Geometry check sheet. Reference: the model listing, model coordinates, mm. Round coordinates to 2 decimals unless told otherwise and drop trailing zeros. One line per question, with ' | ' between items.
Autodesk Inventor part; units mm, degrees
ref_plane "Start Plane" through (20, 0, 0) normal (1, 0, 0) x (0, 1, 0)
ref_plane "End Plane" through (220.5, 0, 0) normal (1, 0, 0) x (0, 1, 0)
ref_plane "XZ Plane" through (0, 0, 0) normal (0, 1, 0) x (-1, 0, 0)
ref_plane "Start Plane" through (20, 0, 0) normal (1, 0, 0) x (0, 1, 0)
ref_plane "End Plane" through (220.5, 0, 0) normal (1, 0, 0) x (0, 1, 0)
sketch "Sketch" plane through (0, 0, 0) normal (1, 0, 0) x (0, 1, 0)
  circle A0 centre (-3.0533, 11.4582) radius 2.1463
  line L0 (2.4543, 4.6976) -> (0.1995, 6.9525)
  arc A1 (1.8616, 3.2667) -> (2.4543, 4.6976) centre (1.8616, 4.1049) ccw
  line L1 (-0.2466, 3.2667) -> (1.8616, 3.2667)
  arc A2 (-0.2466, 3.2667) -> (-0.5514, 2.9619) centre (-0.2466, 2.9619) ccw
  line L2 (-0.5514, 2.2507) -> (-0.5514, 2.9619)
  arc A3 (-0.5514, 2.2507) -> (0.236, 1.4633) centre (0.236, 2.2507) ccw
  line L3 (4.935, 1.4633) -> (0.236, 1.4633)
  arc A4 (4.935, 1.4633) -> (6.9416, 3.4699) centre (4.935, 3.4699) ccw
  line L4 (6.9416, 8.1689) -> (6.9416, 3.4699)
  arc A5 (6.9416, 8.1689) -> (6.1542, 8.9563) centre (6.1542, 8.1689) ccw
  line L5 (5.443, 8.9563) -> (6.1542, 8.9563)
  arc A6 (5.443, 8.9563) -> (5.1382, 8.6515) centre (5.443, 8.6515) ccw
  line L6 (5.1382, 6.5433) -> (5.1382, 8.6515)
  arc A7 (3.7073, 5.9506) -> (5.1382, 6.5433) centre (4.3, 6.5433) ccw
  line L7 (1.4525, 8.2055) -> (3.7073, 5.9506)
  arc A8 (0.5746, 10.3248) -> (1.4525, 8.2055) centre (3.5718, 10.3248) ccw
  line L8 (0.5746, 12.5917) -> (0.5746, 10.3248)
  arc A9 (1.4525, 14.711) -> (0.5746, 12.5917) centre (3.5718, 12.5917) ccw
  line L9 (3.7073, 16.9658) -> (1.4525, 14.711)
  arc A10 (5.1382, 16.3731) -> (3.7073, 16.9658) centre (4.3, 16.3731) ccw
  line L10 (5.1382, 14.2649) -> (5.1382, 16.3731)
  arc A11 (5.1382, 14.2649) -> (5.443, 13.9601) centre (5.443, 14.2649) ccw
  line L11 (6.1542, 13.9601) -> (5.443, 13.9601)
  arc A12 (6.1542, 13.9601) -> (6.9416, 14.7475) centre (6.1542, 14.7475) ccw
  line L12 (6.9416, 19.4465) -> (6.9416, 14.7475)
  arc A13 (6.9416, 19.4465) -> (4.935, 21.4531) centre (4.935, 19.4465) ccw
  line L13 (0.236, 21.4531) -> (4.935, 21.4531)
  arc A14 (0.236, 21.4531) -> (-0.5514, 20.6657) centre (0.236, 20.6657) ccw
  line L14 (-0.5514, 19.9545) -> (-0.5514, 20.6657)
  arc A15 (-0.5514, 19.9545) -> (-0.2466, 19.6497) centre (-0.2466, 19.9545) ccw
  line L15 (1.8616, 19.6497) -> (-0.2466, 19.6497)
  arc A16 (2.4543, 18.2188) -> (1.8616, 19.6497) centre (1.8616, 18.8115) ccw
  line L16 (0.1995, 15.964) -> (2.4543, 18.2188)
  arc A17 (-1.9199, 15.0861) -> (0.1995, 15.964) centre (-1.9199, 18.0833) ccw
  line L17 (-4.1867, 15.0861) -> (-1.9199, 15.0861)
  arc A18 (-6.306, 15.964) -> (-4.1867, 15.0861) centre (-4.1867, 18.0833) ccw
  line L18 (-8.5609, 18.2188) -> (-6.306, 15.964)
  arc A19 (-7.9682, 19.6497) -> (-8.5609, 18.2188) centre (-7.9682, 18.8115) ccw
  line L19 (-5.86, 19.6497) -> (-7.9682, 19.6497)
  arc A20 (-5.86, 19.6497) -> (-5.5552, 19.9545) centre (-5.86, 19.9545) ccw
  line L20 (-5.5552, 20.6657) -> (-5.5552, 19.9545)
  arc A21 (-5.5552, 20.6657) -> (-6.3426, 21.4531) centre (-6.3426, 20.6657) ccw
  line L21 (-11.0416, 21.4531) -> (-6.3426, 21.4531)
  arc A22 (-11.0416, 21.4531) -> (-13.0482, 19.4465) centre (-11.0416, 19.4465) ccw
  line L22 (-13.0482, 14.7475) -> (-13.0482, 19.4465)
  arc A23 (-13.0482, 14.7475) -> (-12.2608, 13.9601) centre (-12.2608, 14.7475) ccw
  line L23 (-11.5496, 13.9601) -> (-12.2608, 13.9601)
  arc A24 (-11.5496, 13.9601) -> (-11.2448, 14.2649) centre (-11.5496, 14.2649) ccw
  line L24 (-11.2448, 16.3731) -> (-11.2448, 14.2649)
  arc A25 (-9.8139, 16.9658) -> (-11.2448, 16.3731) centre (-10.4066, 16.3731) ccw
  line L25 (-7.559, 14.711) -> (-9.8139, 16.9658)
  arc A26 (-6.6812, 12.5917) -> (-7.559, 14.711) centre (-9.6784, 12.5917) ccw
  line L26 (-6.6812, 10.3248) -> (-6.6812, 12.5917)
  arc A27 (-7.559, 8.2055) -> (-6.6812, 10.3248) centre (-9.6784, 10.3248) ccw
  line L27 (-9.8139, 5.9506) -> (-7.559, 8.2055)
  arc A28 (-11.2448, 6.5433) -> (-9.8139, 5.9506) centre (-10.4066, 6.5433) ccw
  line L28 (-11.2448, 8.6515) -> (-11.2448, 6.5433)
  arc A29 (-11.2448, 8.6515) -> (-11.5496, 8.9563) centre (-11.5496, 8.6515) ccw
  line L29 (-12.2608, 8.9563) -> (-11.5496, 8.9563)
  arc A30 (-12.2608, 8.9563) -> (-13.0482, 8.1689) centre (-12.2608, 8.1689) ccw
  line L30 (-13.0482, 3.4699) -> (-13.0482, 8.1689)
  arc A31 (-13.0482, 3.4699) -> (-11.0416, 1.4633) centre (-11.0416, 3.4699) ccw
  line L31 (-6.3426, 1.4633) -> (-11.0416, 1.4633)
  arc A32 (-6.3426, 1.4633) -> (-5.5552, 2.2507) centre (-6.3426, 2.2507) ccw
  line L32 (-5.5552, 2.9619) -> (-5.5552, 2.2507)
  arc A33 (-5.5552, 2.9619) -> (-5.86, 3.2667) centre (-5.86, 2.9619) ccw
  line L33 (-7.9682, 3.2667) -> (-5.86, 3.2667)
  arc A34 (-8.5609, 4.6976) -> (-7.9682, 3.2667) centre (-7.9682, 4.1049) ccw
  line L34 (-6.306, 6.9525) -> (-8.5609, 4.6976)
  arc A35 (-4.1867, 7.8303) -> (-6.306, 6.9525) centre (-4.1867, 4.8331) ccw
  line L35 (-1.9199, 7.8303) -> (-4.1867, 7.8303)
  arc A36 (0.1995, 6.9525) -> (-1.9199, 7.8303) centre (-1.9199, 4.8331) ccw
  point P0 (0, 0)
extrude "Body" add sketch "Sketch" along normal up to surface (200.5 mm away) from surface at 20
sketch "Sketch2" plane through (0, 0, 0) normal (1, 0, 0) x (0, 1, 0)
  line L0 (0, 0) -> (10, 0)
ref_plane "Work Plane3" through (0, 0, 0) normal (0, 0, -1) x (0, 1, 0)
sketch "Sketch3" plane through (0, 0, 0) normal (0, 0, -1) x (0, 1, 0)
  line L0 (-2, 20) -> (12, 20)
  line L1 (-2, 220.5) -> (12, 220.5)
  dimension "d7" = 200.5
equation "\"G_OFFSET_START\" = -20"
equation "\"G_OFFSET_END\" = -20"
equation "\"d2\" = -G_OFFSET_START"
equation "\"d3\" = length + G_OFFSET_END"
equation "\"G_L\" = d7"
properties part number "Generic-1"
(1) Material ranges on line 1 (Z direction, x = 187.5, y = 0.25); line 2 (Z direction, x = 181.5, y = 2); line 3 (Z direction, x = 89, y = 1.75), recorded low to high.
Resolved:
line 1: z = 1.46 to 3.27, 6.9 to 16.01, 19.65 to 21.45 | line 2: z = 1.46 to 3.28, 5.15 to 7.66, 15.26 to 17.76, 19.64 to 21.45 | line 3: z = 1.46 to 3.27, 5.4 to 7.91, 15.01 to 17.51, 19.65 to 21.45
(2) Go/stop test with flat-tipped pins: pin 1 (1.1 mm diameter, centred on x = 136, y = -3.5, fed in from -Z); pin 2 (0.6 mm diameter, centred on x = 152, y = -12, fed in from -Z); pin 3 (1.1 mm diameter, centred on x = 160, z = 11.5, fed in from -Y). Record where each tip stops, or that it passes through.
Resolved:
pin 1: stops at z = 7.83 | pin 2: stops at z = 1.57 | pin 3: stops at y = -6.68
(3) Draft check along Y on faces 1 (the flat face through (119, 3, 1.463)), 2 (the flat face through (119, 6.942, 17)), 3 (the cylindrical face through (118.85, -2.06, 13.36)). Enter one of: +Y half, -Y half, draft (parallel to the pull), parting line (faces both ways), or undercut.
Resolved:
face 1: draft | face 2: +Y half | face 3: undercut
